```python
from build123d import *

# Parameters (mm, degrees)
F0_W     = 960
F0_H     = 640
F1_DEPTH = 160
F3_DEPTH = 160
F5_DEPTH = 120
F7_DEPTH = 420
F9_DEPTH = 160


with BuildPart() as f1:
    # F0 (on Top) → F1 (new body)
    with BuildSketch(Plane.XY):
        with Locations((-431.9713334739, 289.2694023252)):
            Rectangle(F0_W, F0_H)
    extrude(amount=F1_DEPTH)

    # F2 (on face) → F3 (join)
    with BuildSketch(Plane(origin=(-911.9713334739, 0, 0), x_dir=(0, -1, 0), z_dir=(-1, 0, 0))):
        with BuildLine():
            Line((-609.2694023252, 640), (-609.2694023252, 160))
            Line((-609.2694023252, 160), (30.7305976748, 160))
            Line((30.7305976748, 160), (30.7305976748, 320))
            ThreePointArc((30.7305976748, 320), (-62.9952323455, 546.2741699797), (-289.2694023252, 640))
            Line((-289.2694023252, 640), (-609.2694023252, 640))
        make_face()
    extrude(amount=-F3_DEPTH)

    # F4 (on face) → F5 (join)
    with BuildSketch(Plane(origin=(0, 609.2694023252, 0), x_dir=(-1, 0, 0), z_dir=(0, 1, 0))):
        Polygon((-48.0286665261, 160), (351.9713334739, 160), (351.9713334739, 440), align=None)
    extrude(amount=-F5_DEPTH)

    # F6 (on face) → F7 (join)
    with BuildSketch(Plane(origin=(0, 609.2694023252, 0), x_dir=(-1, 0, 0), z_dir=(0, 1, 0))):
        with BuildLine():
            Line((431.9713334739, 440), (351.9713334739, 440))
            Line((351.9713334739, 440), (351.9713334739, 160))
            Line((351.9713334739, 160), (751.9713334739, 160))
            Line((751.9713334739, 160), (751.9713334739, 440))
            Line((751.9713334739, 440), (671.9713334739, 440))
            ThreePointArc((671.9713334739, 440), (551.9713334739, 320), (431.9713334739, 440))
        make_face()
    extrude(amount=-F7_DEPTH)

    # F8 (on face) → F9 (cut)
    with BuildSketch(Plane.XY.offset(160)):
        with BuildLine():
            Line((-151.9713334739, 149.2694023252), (48.0286665261, 149.2694023252))
            Line((48.0286665261, 149.2694023252), (48.0286665261, 309.2694023252))
            Line((48.0286665261, 309.2694023252), (-151.9713334739, 309.2694023252))
            ThreePointArc((-151.9713334739, 309.2694023252), (-231.9713334739, 229.2694023252), (-151.9713334739, 149.2694023252))
        make_face()
    extrude(amount=-F9_DEPTH, mode=Mode.SUBTRACT)


solid = f1.part
```
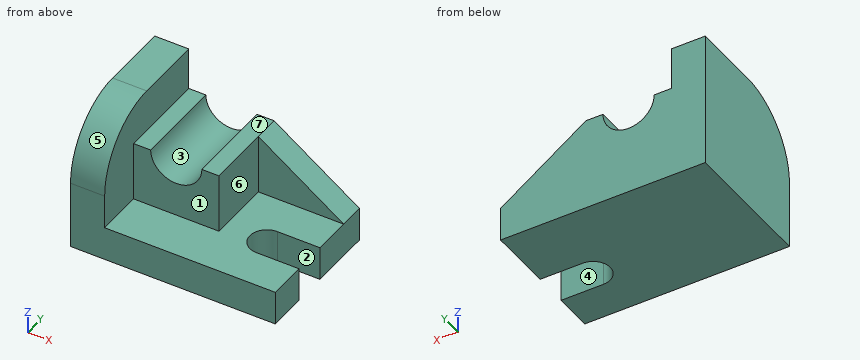
Here's how the part is built. I have some questions about the finished solid (model axes, mm). Face numbers are marked on the shaded views. A direction names the side the tool comes from. Coordinates: 2 decimals unless noted, no trailing zeros. Order: outer loops, then holes, each group sorted by start corner. A loop starts at its lowest first (then second) coordinate and runs counter-clockwise, first axis right, second up.
1) Imagine slicing it at B-B on y = 434.5. List the corners of the cut face in (x, z) for me, and give its area (3 significant figures).
2) Will these pins go through, and if not, where does the flat tip stop? pin 1 (6 mm diameter, centred on x = -591.5, y = 200.5, fed in from +Z); pin 2 (4 mm diameter, centred on x = -370.5, y = 497.5, fed in from +Z).
3) Imagine slicing it at C-C on z = 119.5. List the corners of the cut face in (x, y) for me, and give its area (3 significant figures).
4) Which directions (+Z, -Z, +X, -X, +Y, -Y) give clear straight access to the entire face, cutting with the end or side of a thin tool? Please do the marked faces 5, 6 and 7.
5) We'd pull the mould along Y, two halves only. Please class the marked faces 1, 2, 3 and 4: +Y half, -Y half, draft (parallel to the pull), parting line (faces both ways), or undercut.
6) Imagine slicing it at D-D on x = -405. List the corners of the cut face in (y, z) for me, and give its area (3 significant figures).
7) I need wall thicknesses on line 1 (Y direction, x = -191.5, z = 227.5); line 2 (Y direction, x = -610, z = 288); line 3 (X direction, y = 526.5, z = 463.5). Which ranges of each line are inside material? Lowest first, please.
8) Imagine slicing it at A-A on x = -120.5. List the corners of the cut face in (y, z) for me, and give its area (3 significant figures).
Response values:
1. outline: (-911.97, 0) - (48.03, 0) - (48.03, 160) - (-351.97, 160) - (-351.97, 440) - (-431.97, 440) arc R120 cw to (-671.97, 440) - (-751.97, 440) - (-751.97, 640) - (-911.97, 640) - close
1. area: 320,000 mm2
2. pin 1: stops at z = 327.79
2. pin 2: stops at z = 440
3. outline: (-911.97, -30.73) - (48.03, -30.73) - (48.03, 149.27) - (-151.97, 149.27) arc R80 cw to (-151.97, 309.27) - (48.03, 309.27) - (48.03, 609.27) - (-911.97, 609.27) - close
3. area: 572,000 mm2
4. face 5: +Z, +X, -X, -Y
4. face 6: +Z, +X, -Y
4. face 7: +Z, +X, +Y, -Y
5. face 1: -Y half
5. face 2: undercut
5. face 3: draft
5. face 4: undercut
6. outline: (-30.73, 0) - (609.27, 0) - (609.27, 440) - (189.27, 440) - (189.27, 160) - (-30.73, 160) - close
6. area: 220,000 mm2
7. line 1: y = 489.27 to 609.27
7. line 2: y = 189.27 to 609.27
7. line 3: x = -911.97 to -751.97
8. outline: (-30.73, 0) - (149.27, 0) - (149.27, 160) - (-30.73, 160) - close; (309.27, 0) - (609.27, 0) - (609.27, 277.97) - (489.27, 277.97) - (489.27, 160) - (309.27, 160) - close
8. area: 91,000 mm2
